from build123d import *

# Parameters (mm, degrees)
SKETCH1_R           = 2
BOSS_EXTRUDE1_DEPTH = 1.6
SKETCH1_3_W         = 8.2
SKETCH1_3_H         = 8.2
SKETCH1_3_W_2       = 6.2
SKETCH1_3_H_2       = 6.2
BOSS_EXTRUDE2_DEPTH = 2
BOSS_EXTRUDE3_START = -0.5
SKETCH1_4_W         = 8.2
SKETCH1_4_H         = 8.2
SKETCH1_4_W_2       = 6.2
SKETCH1_4_H_2       = 6.2
SKETCH1_4_R         = 2
BOSS_EXTRUDE3_DEPTH = 0.5
SKETCH3_W           = 5.8
SKETCH3_H           = 5.8
BOSS_EXTRUDE4_DEPTH = 4.5
CHAMFER1_SIZE       = 0.5
CUT_EXTRUDE1_DEPTH  = 0.2


with BuildPart() as part:
    # Sketch1 → Boss-Extrude1 (new body)
    with BuildSketch(Plane(origin=(0, 0, 0), x_dir=(1, 0, 0), z_dir=(0, 1, 0))):
        with Locations(Location((0, 0, 0), (0, 0, 270))):
            Circle(SKETCH1_R)
    extrude(amount=BOSS_EXTRUDE1_DEPTH)



with BuildPart() as body_2:
    # Sketch1_3 → Boss-Extrude2 (new body)
    with BuildSketch(Plane(origin=(0, 0, 0), x_dir=(1, 0, 0), z_dir=(0, 1, 0))):
        Rectangle(SKETCH1_3_W, SKETCH1_3_H)
        Rectangle(SKETCH1_3_W_2, SKETCH1_3_H_2, mode=Mode.SUBTRACT)
    extrude(amount=BOSS_EXTRUDE2_DEPTH)


with BuildPart() as part_1:
    add(part.part)

    add(body_2.part)  # Boss-Extrude3 merges body 2
    # Sketch1_4 → Boss-Extrude3 (add)
    # profile 1 of 3: a face of its own
    with BuildSketch(Plane(origin=(0, 0, 0), x_dir=(1, 0, 0), z_dir=(0, 1, 0)).offset(BOSS_EXTRUDE3_START)):
        Rectangle(SKETCH1_4_W, SKETCH1_4_H)
        Rectangle(SKETCH1_4_W_2, SKETCH1_4_H_2, mode=Mode.SUBTRACT)
    # profile 2 of 3: a face of its own
    with BuildSketch(Plane(origin=(0, 0, 0), x_dir=(1, 0, 0), z_dir=(0, 1, 0)).offset(BOSS_EXTRUDE3_START)):
        Rectangle(SKETCH1_4_W_2, SKETCH1_4_H_2)
        with Locations(Location((0, 0, 0), (0, 0, 270))):
            Circle(SKETCH1_4_R, mode=Mode.SUBTRACT)
    # profile 3 of 3: a face of its own
    with BuildSketch(Plane(origin=(0, 0, 0), x_dir=(1, 0, 0), z_dir=(0, 1, 0)).offset(BOSS_EXTRUDE3_START)):
        with Locations(Location((0, 0, 0), (0, 0, 270))):
            Circle(SKETCH1_4_R)
    extrude(amount=BOSS_EXTRUDE3_DEPTH)

    # Sketch3 → Boss-Extrude4 (add)
    with BuildSketch(Plane.XZ.offset(0.5)):
        Rectangle(SKETCH3_W, SKETCH3_H)
    extrude(amount=BOSS_EXTRUDE4_DEPTH)

    # Chamfer1
    chamfer1_edges = [part_1.edges().sort_by_distance(p)[0] for p in [
        (2.9, -2.75, -2.9),
        (2.9, -2.75, 2.9),
        (-2.9, -2.75, 2.9),
        (-2.9, -2.75, -2.9),
        (-4.1, 0.75, -4.1),
        (4.1, 0.75, -4.1),
        (4.1, 0.75, 4.1),
        (-4.1, 0.75, 4.1),
    ]]
    chamfer(chamfer1_edges, length=CHAMFER1_SIZE)

    # Sketch4 → Cut-Extrude1 (cut)
    with BuildSketch(Plane.XZ.offset(5)):
        with BuildLine():
            Line((-1.040290833, -1.059014553), (-0.744417436, -0.881630739))
            add(Edge.make_bspline(
                [(-0.744417436, -0.881630739), (-0.716899199, -0.927695124), (-0.664175318, -1.015952708), (-0.576223959, -1.135210748), (-0.485091048, -1.236572905), (-0.390101714, -1.319449512), (-0.291835766, -1.384698399), (-0.189651712, -1.430900631), (-0.083893902, -1.459716606), (-0.01192008, -1.463216693), (0.024012051, -1.464964072)],
                knots=[0, 0, 0, 0, 1.272034388, 2.437168799, 3.508375237, 4.49857839, 5.41946034, 6.295179144, 7.148887113, 8, 8, 8, 8], degree=3))
            add(Edge.make_bspline(
                [(0.024012051, -1.464964072), (0.054698912, -1.464109399), (0.115535685, -1.462415009), (0.205097928, -1.446134207), (0.29207973, -1.421122078), (0.374688368, -1.385301147), (0.451783982, -1.341962661), (0.519390678, -1.289616484), (0.577836791, -1.231010278), (0.625645905, -1.165627623), (0.662325941, -1.095310475), (0.690518009, -1.023134523), (0.706163083, -0.947965955), (0.708519836, -0.897355492), (0.709709167, -0.871815034)],
                knots=[0, 0, 0, 0, 1.095163259, 2.171163733, 3.241058638, 4.321873601, 5.38011039, 6.391990106, 7.366004449, 8.327778327, 9.272591725, 10.192022065, 11.087607919, 12, 12, 12, 12], degree=3))
            add(Edge.make_bspline(
                [(0.709709167, -0.871815034), (0.708234856, -0.842674184), (0.705237798, -0.783435095), (0.679906318, -0.696035442), (0.640057071, -0.609542872), (0.603294427, -0.556041606), (0.584208365, -0.528265354)],
                knots=[0, 0, 0, 0, 0.938893495, 1.908633276, 2.914225137, 4, 4, 4, 4], degree=3))
            add(Edge.make_bspline(
                [(0.584208365, -0.528265354), (0.568537751, -0.50821853), (0.535639257, -0.466132732), (0.479081744, -0.403487496), (0.41271563, -0.338869077), (0.338812075, -0.269810021), (0.254678986, -0.199522224), (0.162951472, -0.124653946), (0.061287613, -0.048052369), (-0.010011884, 0.003320197), (-0.04680125, 0.029827595)],
                knots=[0, 0, 0, 0, 0.722233717, 1.516239348, 2.393582979, 3.351407094, 4.387010283, 5.505090956, 6.712668013, 8, 8, 8, 8], degree=3))
            add(Edge.make_bspline(
                [(-0.04680125, 0.029827595), (-0.083625246, 0.056056182), (-0.154029923, 0.106203245), (-0.252488505, 0.180627529), (-0.340532968, 0.248671398), (-0.417771985, 0.31097541), (-0.484171581, 0.367548015), (-0.540254992, 0.417845954), (-0.58459355, 0.463229515), (-0.60924913, 0.492670857), (-0.620318878, 0.505889293)],
                knots=[0, 0, 0, 0, 1.452282411, 2.77665338, 3.964542531, 5.026858415, 5.96415736, 6.766646006, 7.446254459, 8, 8, 8, 8], degree=3))
            add(Edge.make_bspline(
                [(-0.620318878, 0.505889293), (-0.635791423, 0.52649033), (-0.66622026, 0.567005034), (-0.706386266, 0.630329892), (-0.740525428, 0.695153157), (-0.76728776, 0.761649022), (-0.789823979, 0.828883951), (-0.80498191, 0.897735196), (-0.814473307, 0.967893815), (-0.815445293, 1.015107315), (-0.815931859, 1.038741857)],
                knots=[0, 0, 0, 0, 1.068054152, 2.10047183, 3.106115577, 4.101338837, 5.06977816, 6.043150881, 7.020423561, 8, 8, 8, 8], degree=3))
            add(Edge.make_bspline(
                [(-0.815931859, 1.038741857), (-0.81462665, 1.075771632), (-0.81204413, 1.149039696), (-0.790203613, 1.256070526), (-0.755730719, 1.358256943), (-0.707435831, 1.454587277), (-0.645178478, 1.542553258), (-0.573132504, 1.623166745), (-0.487321018, 1.690935327), (-0.393168394, 1.750147386), (-0.290112022, 1.796493311), (-0.182121119, 1.831454291), (-0.069024047, 1.851263549), (0.007579088, 1.854106314), (0.046447949, 1.855548749)],
                knots=[0, 0, 0, 0, 1.005424448, 1.989358655, 2.955360095, 3.929531133, 4.905563448, 5.876582895, 6.856512386, 7.866279853, 8.892233794, 9.918561126, 10.94386622, 12, 12, 12, 12], degree=3))
            add(Edge.make_bspline(
                [(0.046447949, 1.855548749), (0.087692049, 1.854126197), (0.169713401, 1.851297196), (0.290362616, 1.826699664), (0.406523333, 1.785998993), (0.499966598, 1.739810335), (0.573099359, 1.693678919), (0.628872092, 1.651659095), (0.685389543, 1.603283986), (0.743107597, 1.54842474), (0.801048257, 1.486577989), (0.860071709, 1.4181673), (0.920315978, 1.343610744), (0.959071838, 1.290386243), (0.978939936, 1.263100832)],
                knots=[0, 0, 0, 0, 1.286793592, 2.559021753, 3.825965368, 5.121522368, 5.803751409, 6.523245864, 7.299691795, 8.125521123, 9.008227632, 9.944561021, 10.946284179, 12, 12, 12, 12], degree=3))
            Line((0.978939936, 1.263100832), (0.694985609, 1.047856441))
            add(Edge.make_bspline(
                [(0.694985609, 1.047856441), (0.677839677, 1.069945131), (0.644820619, 1.112482784), (0.594691133, 1.1720541), (0.547442485, 1.22647058), (0.500892085, 1.273735708), (0.457498453, 1.316437841), (0.415381411, 1.352997598), (0.37514706, 1.383773193), (0.324430149, 1.416616753), (0.260712431, 1.449173257), (0.180727895, 1.476722335), (0.09714162, 1.493277397), (0.040211988, 1.495466284), (0.011391859, 1.49657439)],
                knots=[0, 0, 0, 0, 1.181633172, 2.275549214, 3.290209073, 4.226197932, 5.078386478, 5.862611352, 6.581680152, 7.217281963, 8.414376989, 9.595101626, 10.782541182, 12, 12, 12, 12], degree=3))
            add(Edge.make_bspline(
                [(0.011391859, 1.49657439), (-0.024764663, 1.49536269), (-0.094489111, 1.49302604), (-0.193479347, 1.467506055), (-0.282573272, 1.427324195), (-0.359125837, 1.371009217), (-0.422862814, 1.304288224), (-0.468968273, 1.227509369), (-0.496718437, 1.142726966), (-0.500104717, 1.08358531), (-0.501829295, 1.053465415)],
                knots=[0, 0, 0, 0, 1.14458467, 2.207223713, 3.21896685, 4.227309161, 5.202851033, 6.127160689, 7.046193047, 8, 8, 8, 8], degree=3))
            add(Edge.make_bspline(
                [(-0.501829295, 1.053465415), (-0.501436168, 1.034713937), (-0.500649272, 0.997180317), (-0.489674474, 0.941728895), (-0.475575145, 0.886417556), (-0.453232514, 0.831494973), (-0.42238721, 0.776000614), (-0.381882034, 0.718978876), (-0.330868722, 0.659927168), (-0.29179171, 0.621519794), (-0.271160224, 0.601241857)],
                knots=[0, 0, 0, 0, 0.858281714, 1.717966888, 2.583508476, 3.4729293, 4.427298488, 5.488583878, 6.674047936, 8, 8, 8, 8], degree=3))
            add(Edge.make_bspline(
                [(-0.271160224, 0.601241857), (-0.263498852, 0.594404832), (-0.245297185, 0.578161623), (-0.212021259, 0.551569343), (-0.168078461, 0.51876657), (-0.11461626, 0.478179254), (-0.050648898, 0.431097792), (0.023830658, 0.37812418), (0.107992191, 0.317538721), (0.167714107, 0.27518118), (0.1992925, 0.252784325)],
                knots=[0, 0, 0, 0, 0.420754252, 0.999615792, 1.744751191, 2.668019286, 3.750313428, 4.999500688, 6.413464383, 8, 8, 8, 8], degree=3))
            add(Edge.make_bspline(
                [(0.1992925, 0.252784325), (0.237278413, 0.225142966), (0.31083287, 0.171619304), (0.41549045, 0.091203624), (0.510384258, 0.012555856), (0.595847461, -0.063821752), (0.67272437, -0.137349845), (0.74016209, -0.208913025), (0.798847771, -0.277998598), (0.862026989, -0.366571173), (0.926584809, -0.475352258), (0.982026316, -0.608630496), (1.016984664, -0.742426817), (1.021556179, -0.832353653), (1.023811731, -0.876722886)],
                knots=[0, 0, 0, 0, 1.163667725, 2.253281268, 3.268753668, 4.215851969, 5.092017293, 5.902905408, 6.650798638, 7.335211899, 8.59617414, 9.77448103, 10.901945474, 12, 12, 12, 12], degree=3))
            add(Edge.make_bspline(
                [(1.023811731, -0.876722886), (1.023154593, -0.908101251), (1.021853078, -0.970248635), (1.006892164, -1.061503712), (0.984972499, -1.150134581), (0.951935265, -1.235045694), (0.911612106, -1.317790456), (0.860445859, -1.396198357), (0.801138174, -1.472004755), (0.733104409, -1.543188247), (0.658658507, -1.608534443), (0.579974812, -1.666663504), (0.496924539, -1.715131828), (0.409958222, -1.75468267), (0.319055886, -1.785616187), (0.224248102, -1.808029056), (0.125378591, -1.821784767), (0.058178109, -1.823212529), (0.024012051, -1.823938431)],
                knots=[0, 0, 0, 0, 0.983748083, 1.948392443, 2.894712957, 3.844097841, 4.80183111, 5.778335162, 6.776009319, 7.81870978, 8.863265674, 9.881300176, 10.883814829, 11.87499822, 12.874611388, 13.892143829, 14.928324115, 16, 16, 16, 16], degree=3))
            add(Edge.make_bspline(
                [(0.024012051, -1.823938431), (-0.002423292, -1.823427249), (-0.054961052, -1.822411324), (-0.132670534, -1.813430044), (-0.208810123, -1.80072294), (-0.282424405, -1.78054887), (-0.354461816, -1.756071893), (-0.424609051, -1.72593356), (-0.492900105, -1.689816359), (-0.559717688, -1.648521334), (-0.624891862, -1.60046359), (-0.68781133, -1.544490093), (-0.750540516, -1.482144588), (-0.811227912, -1.411734025), (-0.871101056, -1.334395942), (-0.928979466, -1.249406759), (-0.986061184, -1.157229405), (-1.021876651, -1.092364319), (-1.040290833, -1.059014553)],
                knots=[0, 0, 0, 0, 0.915332311, 1.819136955, 2.706846663, 3.586547465, 4.459518054, 5.340707479, 6.227863349, 7.133153174, 8.059268498, 9.028702269, 10.047606654, 11.120612155, 12.245963614, 13.433783089, 14.680604001, 16, 16, 16, 16], degree=3))
        make_face()
    extrude(amount=-CUT_EXTRUDE1_DEPTH, mode=Mode.SUBTRACT)


solid = part_1.part
Verification items for the finished model (mm, model axes). A direction names the side the tool comes from. Give positions to 0.01 mm unless a question says otherwise; leave off trailing zeros. Loops run counter-clockwise (first coordinate to the right, second up) from the corner with the lowest first, then second, coordinate; pieces in that order, holes last.
1) Sectioned sample at C-C, the plane y = -2.75. Enter the section's corners in (x, z).
2) Sectioned sample at D-D, the plane x = 2.75. Enter the section's corners in (y, z), then the cut area to 4 significant figures.
3) Thickness scan on line 1 along X through (y, z) = (1.5, -3); line 2 along Z through (x, y) = (1, 0.75); line 3 along Y through (x, z) = (-0.5, -0.75). Record the ranges inside material, lowest first.
4) Depth check by flat-ended pin: pin 1 Ø1.3 at (x, y) = (0, -3.5) entering from -Z; pin 2 Ø2 at (y, z) = (-3.5, 1) entering from +X; pin 3 Ø4.5 at (x, z) = (-0.5, 0.5) entering from +Y. Enter the tip coordinate at first touch or a pass-through.
5) Sectioned sample at A-A, the plane y = 1. Enter the section's corners in (x, z), then the cut area to 3 significant figures.
6) Sectioned sample at B-B, the plane z = -2.25. Enter the section's corners in (x, y), then the cut area to 3 significant figures.
7) Draft check along Z on faces 5 (the flat face through (0, -5, -1)), 6 (the flat face through (-1, 0, -2)), 7 (the flat face through (0, 1, 4.1)), 8 (the flat face through (0, 1, 3.1)). Enter one of: pulls with the +Z half, pulls with the -Z half, needs draft (parallel to the pull), parting line crosses it, or undercut.
8) Set-up check for faces 1 (the flat face through (-2.9, -3, 0)), 2 (the flat face through (-3.1, 1, 0)), 3 (the flat face through (0.07, -4.8, 0.16)), 4 (the flat face through (0, -3, -2.9)): record each of +Z, -Z, +X, -X, +Y, -Y from which the full face is reachable in a straight line by a thin tool's end or side.
Answers:
1. outline: (-2.9, -2.4) - (-2.4, -2.9) - (2.4, -2.9) - (2.9, -2.4) - (2.9, 2.4) - (2.4, 2.9) - (-2.4, 2.9) - (-2.9, 2.4) - close
2. outline: (-5, -2.55) - (-0.5, -2.55) - (-0.5, -4.1) - (2, -4.1) - (2, -3.1) - (0, -3.1) - (0, 3.1) - (2, 3.1) - (2, 4.1) - (-0.5, 4.1) - (-0.5, 2.55) - (-5, 2.55) - close
2. area: 31.05 mm2
3. line 1: x = -4.1 to -3.1, 3.1 to 4.1
3. line 2: z = -4.1 to -3.1, -1.73 to 1.73, 3.1 to 4.1
3. line 3: y = -5 to 1.6
4. pin 1: stops at z = -2.9
4. pin 2: stops at x = 2.9
4. pin 3: stops at y = 1.6
5. outline: (-4.1, -3.6) - (-3.6, -4.1) - (3.6, -4.1) - (4.1, -3.6) - (4.1, 3.6) - (3.6, 4.1) - (-3.6, 4.1) - (-4.1, 3.6) - close; circle Ø4 at (0, 0); hole (-3.1, -3.1) - (3.1, -3.1) - (3.1, 3.1) - (-3.1, 3.1) - close
5. area: 40.9 mm2
6. outline: (-4.1, -0.5) - (-2.9, -0.5) - (-2.9, -5) - (2.9, -5) - (2.9, -0.5) - (4.1, -0.5) - (4.1, 2) - (3.1, 2) - (3.1, 0) - (-3.1, 0) - (-3.1, 2) - (-4.1, 2) - close
6. area: 34.2 mm2
7. face 5: needs draft
7. face 6: undercut
7. face 7: pulls with the +Z half
7. face 8: undercut
8. face 1: +Z, -Z, -X, -Y
8. face 2: +Y
8. face 3: -Y
8. face 4: -Z, +X, -X, -Y
